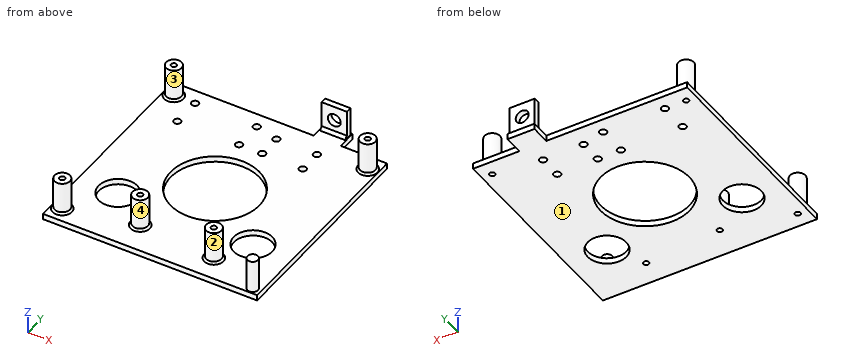
```python
from build123d import *

# Parameters (mm, degrees)
SKETCH001_R                          = 4
SKETCH001_R_2                        = 1.4
SKETCH001_R_3                        = 2.75
EXTRUDE001_DEPTH                     = 20
SKETCH002_AS_DRAWN_W                 = 13
SKETCH002_AS_DRAWN_H                 = 15
SKETCH002_AS_DRAWN_R                 = 3.35
EXTRUDE002_DEPTH                     = 3
EXTRUDE002_ONTO_SKETCH002_ROLL_ANGLE = 90
SKETCH_R                             = 1.9
SKETCH_R_2                           = 10
SKETCH_R_3                           = 23
SKETCH_R_4                           = 1.85
EXTRUDE_DEPTH                        = 3
CHAMFER_1_SIZE                       = 1.5
CHAMFER_2_SIZE                       = 1


with BuildPart() as extrude001:
    # Sketch001 → Extrude001 (new body)
    with BuildSketch(Plane.XY):
        with Locations((-50.25, -47.25)):
            Circle(SKETCH001_R)
        with Locations((-50.25, -47.25)):
            Circle(SKETCH001_R_2, mode=Mode.SUBTRACT)
        with Locations((50.25, 47.25)):
            Circle(SKETCH001_R)
        with Locations((50.25, 47.25)):
            Circle(SKETCH001_R_2, mode=Mode.SUBTRACT)
        with Locations((-50.25, 47.25)):
            Circle(SKETCH001_R)
        with Locations((-50.25, 47.25)):
            Circle(SKETCH001_R_2, mode=Mode.SUBTRACT)
        with Locations((25.25, -42.25)):
            Circle(SKETCH001_R)
        with Locations((25.25, -42.25)):
            Circle(SKETCH001_R_2, mode=Mode.SUBTRACT)
        with Locations((51.25, -51.75)):
            Circle(SKETCH001_R_3)
        with Locations((-14.75, -39.25)):
            Circle(SKETCH001_R)
        with Locations((-14.75, -39.25)):
            Circle(SKETCH001_R_2, mode=Mode.SUBTRACT)
    extrude(amount=EXTRUDE001_DEPTH)


with BuildPart() as extrude002:
    # Sketch002 as drawn → Extrude002 (new)
    with BuildSketch(Plane.XY):
        with Locations((36.5, 7.5)):
            Rectangle(SKETCH002_AS_DRAWN_W, SKETCH002_AS_DRAWN_H)
        with Locations((36.5, 7.5)):
            Circle(SKETCH002_AS_DRAWN_R, mode=Mode.SUBTRACT)
    extrude(amount=-EXTRUDE002_DEPTH)


with BuildPart() as extrude002_1:
    # Extrude002 onto Sketch002 roll: moved
    add(extrude002.part.rotate(Axis((0, 0, 0), (1, 0, 0)), EXTRUDE002_ONTO_SKETCH002_ROLL_ANGLE))


with BuildPart() as extrude002_2:
    # Extrude002 onto Sketch002 placement: moved
    add(extrude002_1.part)


with BuildPart() as extrude002_3:
    # Extrude002 placement: moved
    add(extrude002_2.part.moved(Location((-12, 61, 3))))


with BuildPart() as chamfer_body:
    # Sketch → Extrude (new body)
    with BuildSketch(Plane.XY):
        Polygon((55.5, 55), (55.5, -55), (-55.5, -55), (-55.5, 55), (17.5, 55), (17.5, 65), (31.5, 65), (31.5, 55), align=None)
        with Locations((-50.25, -47.25)):
            Circle(SKETCH_R, mode=Mode.SUBTRACT)
        with Locations((35, -25)):
            Circle(SKETCH_R_2, mode=Mode.SUBTRACT)
        with Locations((-35, -25)):
            Circle(SKETCH_R_2, mode=Mode.SUBTRACT)
        Circle(SKETCH_R_3, mode=Mode.SUBTRACT)
        with Locations((-39.25, 47.25)):
            Circle(SKETCH_R_4, mode=Mode.SUBTRACT)
        with Locations((-7.25, 47.25)):
            Circle(SKETCH_R_4, mode=Mode.SUBTRACT)
        with Locations((-39.25, 32.25)):
            Circle(SKETCH_R_4, mode=Mode.SUBTRACT)
        with Locations((-7.25, 32.25)):
            Circle(SKETCH_R_4, mode=Mode.SUBTRACT)
        with Locations((4.75, 44.25)):
            Circle(SKETCH_R_4, mode=Mode.SUBTRACT)
        with Locations((25.75, 44.25)):
            Circle(SKETCH_R_4, mode=Mode.SUBTRACT)
        with Locations((4.75, 32.25)):
            Circle(SKETCH_R_4, mode=Mode.SUBTRACT)
        with Locations((25.75, 32.25)):
            Circle(SKETCH_R_4, mode=Mode.SUBTRACT)
        with Locations((50.25, 47.25)):
            Circle(SKETCH_R, mode=Mode.SUBTRACT)
        with Locations((-50.25, 47.25)):
            Circle(SKETCH_R, mode=Mode.SUBTRACT)
        with Locations((25.25, -42.25)):
            Circle(SKETCH_R, mode=Mode.SUBTRACT)
        with Locations((-14.75, -39.25)):
            Circle(SKETCH_R, mode=Mode.SUBTRACT)
    extrude(amount=EXTRUDE_DEPTH)

    # Fusion: union Extrude001, Extrude002
    add(extrude001.part)
    add(extrude002_3.part)

    # Chamfer 1
    chamfer_1_edges = [chamfer_body.edges().sort_by_distance(p)[0] for p in [
        (24.5, 61, 3),
    ]]
    chamfer(chamfer_1_edges, length=CHAMFER_1_SIZE)

    # Chamfer 2
    chamfer_2_edges = [chamfer_body.edges().sort_by_distance(p)[0] for p in [
        (46.25, 47.25, 3),
        (21.25, -42.25, 3),
        (-18.75, -39.25, 3),
        (-54.25, -47.25, 3),
        (-54.25, 47.25, 3),
    ]]
    chamfer(chamfer_2_edges, length=CHAMFER_2_SIZE)


solid = chamfer_body.part
```
Source: CAD feature listing. Evaluate the final solid. Frame: model axes, mm. Face numbers are marked on the shaded views. Coordinates: 2 decimals unless noted, no trailing zeros. Write each loop counter-clockwise with the first axis right and the second up, starting at its lowest first coordinate (ties: lowest second). Pieces come first, ordered by that corner, then holes. Notation, with made-up numbers: (-15.75, -1) - (13.25, -1) arc R28 cw to (13.25, 18) - close; hole circle Ø8 at (-9, 6). An arc over 180 degrees is marked (long way). Answer as a JSON object with one key per item and string values.
Q1. Draft query along Y for the marked faces 1, 2, 3 and 4. Return one class per face: released by +Y, released by -Y, zero draft, split by the parting line, or undercut.
Ans:
{"face 1": "zero draft", "face 2": "undercut", "face 3": "undercut", "face 4": "split by the parting line"}
Q2. Section query D-D, the plane y = 16.5. Output: boundary loops of the cut face in (x, z), plus the area to 3 significant figures.
Ans:
{"outline": "(-55.5, 0) - (-16.02, 0) - (-16.02, 3) - (-55.5, 3) - close; (16.02, 0) - (55.5, 0) - (55.5, 3) - (16.02, 3) - close", "area": "237 mm2"}
Q3. First-contact query: pin 1 Ø6.5 at (x, z) = (25, 11.5) entering from +Y; pin 2 Ø1.5 at (x, z) = (-37, 1) entering from +Y; pin 3 Ø6 at (x, z) = (24.5, 10.5) entering from -Y. Flat tips, straight axial feed; report the tip coordinate or a pass-through.
Ans:
{"pin 1": "stops at y = 64", "pin 2": "stops at y = 55", "pin 3": "stops at y = -46.25"}
Q4. Section query A-A, the plane y = 32.25. Output: boundary loops of the cut face in (x, z).
Ans:
{"outline": "(-55.5, 0) - (-41.1, 0) - (-41.1, 3) - (-55.5, 3) - close; (-37.4, 0) - (-9.1, 0) - (-9.1, 3) - (-37.4, 3) - close; (-5.4, 0) - (2.9, 0) - (2.9, 3) - (-5.4, 3) - close; (6.6, 0) - (23.9, 0) - (23.9, 3) - (6.6, 3) - close; (27.6, 0) - (55.5, 0) - (55.5, 3) - (27.6, 3) - close"}
Q5. Material intervals for line 1 (Y direction, x = -50.25, z = 4.25); line 2 (Y direction, x = -35, z = 1.4); line 3 (Y direction, x = -14.75, z = 6.5), sorted ascending. Write a range as [from, to].
Ans:
{"line 1": "y = [-51.25, -48.65], [-45.85, -43.25], [43.25, 45.85], [48.65, 51.25]", "line 2": "y = [-55, -35], [-15, 55]", "line 3": "y = [-43.25, -40.65], [-37.85, -35.25]"}
Q6. Section query C-C, the plane x = 4.75. Output: boundary loops of the cut face in (y, z), plus the area to 3 significant figures.
Ans:
{"outline": "(-55, 0) - (-22.5, 0) - (-22.5, 3) - (-55, 3) - close; (22.5, 0) - (30.4, 0) - (30.4, 3) - (22.5, 3) - close; (34.1, 0) - (42.4, 0) - (42.4, 3) - (34.1, 3) - close; (46.1, 0) - (55, 0) - (55, 3) - (46.1, 3) - close", "area": "173 mm2"}
Q7. Section query B-B, the plane z = 9. State how many separate pieces and enclosed holes the cut face has, plus the area to 3 significant figures.
Ans:
{"separate pieces": "8", "enclosed holes": "5", "area": "265 mm2"}
